Design review of the part built by this model. Coordinates are the model's own, in mm. Coordinates: 2 decimals unless noted, no trailing zeros. Write each loop counter-clockwise with the first axis right and the second up, starting at its lowest first coordinate (ties: lowest second). Pieces come first, ordered by that corner, then holes. Notation, with made-up numbers: (-25, 51) - (29, 51) arc R20 ccw to (29, 86) - close; hole circle Ø3 at (68.25, 61). An arc over 180 degrees is marked (long way). Answer as CSV lines item,"result". Start each with the question number.
Q1. We need section B-B (y = 30). Write out the cut boundary in (x, z).
Q2. For line 1 along X through (y, z) = (37, 0.15); line 2 along Y through (x, z) = (-1, 0.1); line 3 along Y through (x, z) = (16.5, 0.15), list the stretches that pass through material, from the lowest coordinate up. Write a range as [from, to].
Q3. We need section A-A (z = 0.1). Write out the cut boundary in (x, y), plus the area to 3 significant figures.
Q4. We need section C-C (x = -3). Write out the cut boundary in (y, z), plus the area to 4 significant figures.
from build123d import *

# Parameters (mm, degrees)
F1_DEPTH = 0.2


with BuildPart() as f1:
    # F0 (on Top) → F1 (new body)
    with BuildSketch(Plane.XY):
        with BuildLine():
            Line((-18.75, 37.5), (-37.5, 37.5))
            Line((-37.5, 37.5), (-37.5, -37.5))
            Line((-37.5, -37.5), (37.5, -37.5))
            Line((37.5, -37.5), (37.5, -26.5165042945))
            ThreePointArc((37.5, -26.5165042945), (10.9834957055, 0), (37.5, 26.5165042945))
            Line((37.5, 26.5165042945), (37.5, 37.5))
            Line((37.5, 37.5), (18.75, 37.5))
            Line((18.75, 37.5), (-18.75, 37.5))
        make_face()
        Polygon((0, 56.25), (-18.75, 37.5), (18.75, 37.5), align=None)
        with BuildLine():
            ThreePointArc((37.5, 26.5165042945), (10.9834957055, 0), (37.5, -26.5165042945))
            Line((37.5, -26.5165042945), (37.5, 26.5165042945))
        make_face()
        with BuildLine():
            Line((37.5, 26.5165042945), (37.5, -26.5165042945))
            ThreePointArc((37.5, -26.5165042945), (56.25, -18.75), (64.0165042945, 0))
            ThreePointArc((64.0165042945, 0), (56.25, 18.75), (37.5, 26.5165042945))
        make_face()
    extrude(amount=F1_DEPTH)


solid = f1.part
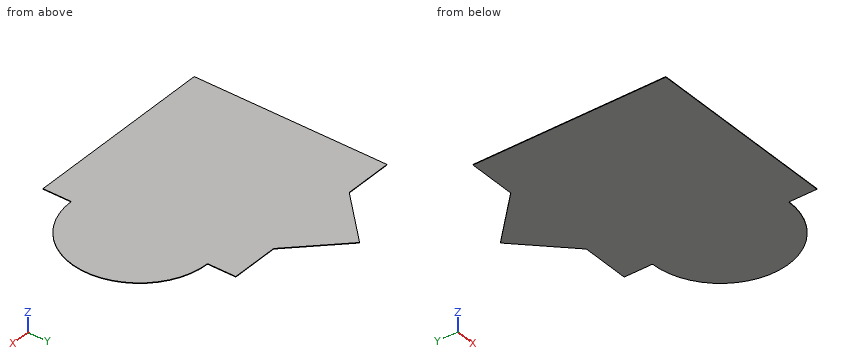
Results list:
1,outline,"(-37.5, 0) - (37.5, 0) - (37.5, 0.2) - (-37.5, 0.2) - close"
2,line 1,"x = [-37.5, 37.5]"
2,line 2,"y = [-37.5, 55.25]"
2,line 3,"y = [-37.5, 39.75]"
3,outline,"(-37.5, -37.5) - (37.5, -37.5) - (37.5, -26.52) arc R26.52 ccw to (37.5, 26.52) - (37.5, 37.5) - (18.75, 37.5) - (0, 56.25) - (-18.75, 37.5) - (-37.5, 37.5) - close"
3,area,"7,080 mm2"
4,outline,"(-37.5, 0) - (53.25, 0) - (53.25, 0.2) - (-37.5, 0.2) - close"
4,area,"18.15 mm2"
